Design review of the part built by this model. Coordinates are the model's own, in mm. Face numbers are marked on the shaded views. A direction names the side the tool comes from. Give positions to 0.01 mm unless a question says otherwise; leave off trailing zeros. Order: outer loops, then holes, each group sorted by start corner. A loop starts at its lowest first (then second) coordinate and runs counter-clockwise, first axis right, second up. Notation, with made-up numbers: (-20, 45) -> (10, 45) arc R22 cw to (10, 55) -> close; hole circle Ø4 at (-3.5, 62.25). An arc over 180 degrees is marked (long way). One line per item, written item: value. Start each with the question number.
1) Consider section B-B (z = -21.5). State the section outline as (x, y) points, plus the area to 3 significant figures.
2) Tool access review of the marked faces 1, 2 and 3: name each direction out of +Z, -Z, +X, -X, +Y, -Y from which nothing blocks a thin tool from reaching the whole face with its end or side.
3) Consider section A-A (x = 0). State how many separate pieces and enclosed holes the cut face has, plus the area to 3 significant figures.
4) Wall thickness on line 1 along Z through (x, y) = (0, -8); line 2 along X through (y, z) = (-10.5, 6); line 3 along X through (y, z) = (-0.75, -7): over which ranges is each line inside the solid? List them lowest first. Write a range as from..to.
5) The part is to be moulded in two halves that separate along Z. For the marked faces 4 and 5, say which applies: released by +Z, released by -Z, zero draft, split by the parting line, or undercut.
6) Consider section D-D (z = 20.5). State the section outline as (x, y) points.
7) For pin 1 (3 mm diameter, centred on y = -11.5, z = 38.5, fed in from +X); pin 2 (5 mm diameter, centred on y = -2.5, z = 47.5, fed in from +X); pin 3 (3 mm diameter, centred on y = -8, z = -30, fed in from -X), all flat-tipped, find the tip position at first contact; note any pin that passes through.
from build123d import *

# Parameters (mm, degrees)
F0_R     = 10.16
F0_R_2   = 6.35
F1_DEPTH = 12.7


with BuildPart() as f1:
    # F0 (on Front) → F1 (new body)
    with BuildSketch(Plane.XZ):
        with BuildLine():
            ThreePointArc((-22.5764605638, 22.324110921), (0, 31.75), (22.5764605638, 22.324110921))
            Line((22.5764605638, 22.324110921), (55.7279327263, 33.6904105914))
            add(Edge.make_bspline(
                [(-53.578904017, 35.5630292681), (-33.5322332568, 70.2029654889), (46.3976245244, 63.5476266624), (55.7279327263, 33.6904105914)],
                knots=[0, 0, 0, 0, 109.3228761949, 109.3228761949, 109.3228761949, 109.3228761949], degree=3))
            Line((-53.578904017, 35.5630292681), (-22.5764605638, 22.324110921))
        make_face()
        with BuildLine():
            ThreePointArc((17.7535295726, -26.3225129445), (28.0333467849, -14.9061721456), (31.75, 0))
            ThreePointArc((31.75, 0), (29.3672021386, 12.067723006), (22.5764605638, 22.324110921))
            ThreePointArc((22.5764605638, 22.324110921), (0, 31.75), (-22.5764605638, 22.324110921))
            ThreePointArc((-22.5764605638, 22.324110921), (-31.6476270633, -2.5475873414), (-18.7147767568, -25.6479946769))
            ThreePointArc((-18.7147767568, -25.6479946769), (-0.5871479887, -31.7445705159), (17.7535295726, -26.3225129445))
        make_face()
        Circle(F0_R, mode=Mode.SUBTRACT)
        with BuildLine():
            add(Edge.make_bspline(
                [(-18.7147767568, -25.6479946769), (-18.9355896144, -33.2121243406), (-19.321526262, -49.686071611), (16.9001065861, -52.1663001494), (17.9694969141, -34.8175484735), (17.7535295726, -26.3225129445)],
                knots=[0, 0, 0, 0, 0.3182872314, 0.6721361216, 1, 1, 1, 1], degree=3))
            ThreePointArc((17.7535295726, -26.3225129445), (-0.5871479887, -31.7445705159), (-18.7147767568, -25.6479946769))
        make_face()
        with Locations((0, -40.6298153102)):
            Circle(F0_R_2, mode=Mode.SUBTRACT)
    extrude(amount=F1_DEPTH)


solid = f1.part
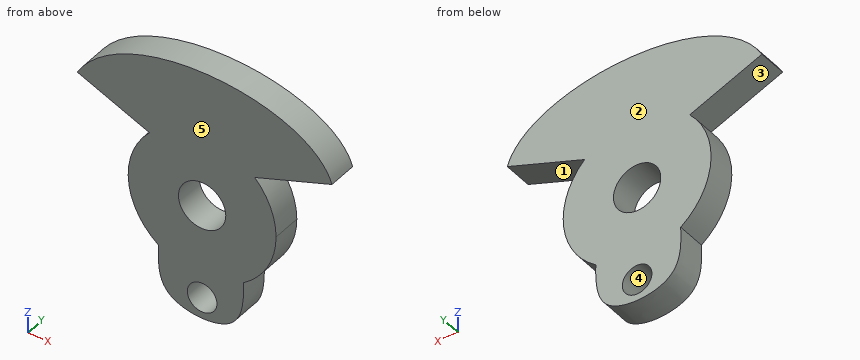
Checked values:
1. outline: (-23.36, -12.7) -> (23.36, -12.7) -> (23.36, 0) -> (-23.36, 0) -> close
1. area: 593 mm^2
2. face 1: +X, +Y, -Y
2. face 2: +Z, -Z, +X, -X, +Y
2. face 3: -X, +Y, -Y
3. separate pieces: 3
3. enclosed holes: 0
3. area: 962 mm^2
4. line 1: z = -49.82..-46.98, -34.28..-10.16, 10.16..58.92
4. line 2: x = -31.18..-8.2, 8.2..31.18
4. line 3: x = -30.97..-7.36, 7.36..30.97
5. face 4: undercut
5. face 5: zero draft
6. outline: (-24.24, -12.7) -> (24.24, -12.7) -> (24.24, 0) -> (-24.24, 0) -> close
7. pin 1: stops at x = 54.36
7. pin 2: stops at x = 47.8
7. pin 3: stops at x = -18.8
